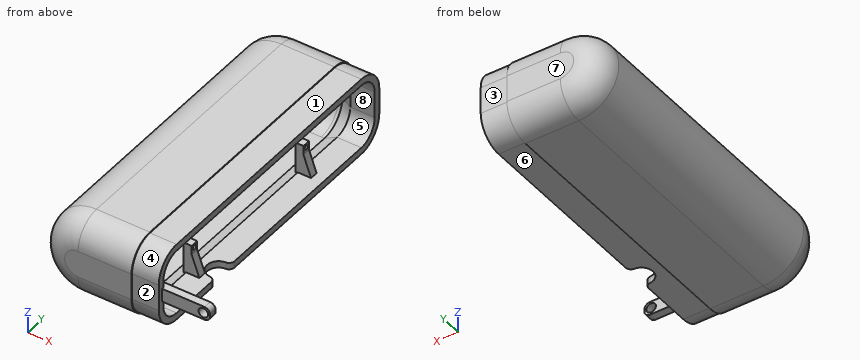
```python
from build123d import *
from OCP.BRepFilletAPI import BRepFilletAPI_MakeChamfer

# Parameters (mm, degrees)
BOSS_EXTRUDE1_DEPTH      = 76.2
FILLET1_R                = 12.7
SHELL1_T                 = -0.4
EXTRUDE_THIN1_DEPTH      = 12.7
EXTRUDE_THIN1_DEPTH_BACK = 6.35
CHAMFER1_SIZE            = 7.46
CHAMFER1_SIZE_2          = 3.96655236
SKETCH6_W                = 17.539309582
SKETCH6_H                = 3.81
SKETCH6_R                = 1.054294776
BOSS_EXTRUDE3_DEPTH      = 3.81
CHAMFER2_SIZE            = 10
CHAMFER2_SIZE2           = 3.639702343
SKETCH7_W                = 33.02
SKETCH7_H                = 6.35
BOSS_EXTRUDE4_DEPTH      = 3.81
CHAMFER3_SIZE            = 3.81
CHAMFER3_SIZE_2          = 4.231433681
SKETCH8_R                = 2.25
CUT_EXTRUDE1_DEPTH       = 160.403972974
FILLET2_R                = 2.54
SKETCH9_R                = 5.461
CUT_EXTRUDE2_DEPTH       = 104.511048806
FILLET3_R                = 2.54


with BuildPart() as part:
    # Sketch1 → Boss-Extrude1 (new, symmetric)
    with BuildSketch(Plane(origin=(0, 0, 0), x_dir=(1, 0, 0), z_dir=(0, 1, 0))):
        with BuildLine():
            Line((0, -19.05), (25.4, -19.05))
            Line((25.4, -19.05), (25.4, 19.05))
            Line((25.4, 19.05), (0, 19.05))
            ThreePointArc((0, 19.05), (-19.05, 0), (0, -19.05))
        make_face()
    extrude(amount=BOSS_EXTRUDE1_DEPTH, both=True)

    # Fillet1
    fillet1_edges = [part.edges().sort_by_distance(p)[0] for p in [
        (12.7, 76.2, -19.05),
        (-19.05, 76.2, 0),
        (12.7, -76.2, -19.05),
        (12.7, -76.2, 19.05),
        (-19.05, -76.2, 0),
        (12.7, 76.2, 19.05),
    ]]
    fillet(fillet1_edges, radius=FILLET1_R)

    # Shell1
    shell1_openings = [part.faces().sort_by_distance(p)[0] for p in [
        (25.4, 0, 0),
    ]]
    offset(amount=SHELL1_T, openings=shell1_openings, kind=Kind.INTERSECTION)

    # Sketch4 → Extrude-Thin1 (add, two sides: drawn at the far end of the back side and taken through both)
    with BuildSketch(Plane(origin=(25.4, 0, 0), x_dir=(0, 0, -1), z_dir=(1, 0, 0)).offset(-EXTRUDE_THIN1_DEPTH_BACK)):
        with BuildLine():
            Line((18.65, 63.5), (18.65, -63.5))
            ThreePointArc((18.65, -63.5), (15.047413409, -72.197413409), (6.35, -75.8))
            Line((6.35, -75.8), (-6.35, -75.8))
            ThreePointArc((-6.35, -75.8), (-15.047413409, -72.197413409), (-18.65, -63.5))
            Line((-18.65, -63.5), (-18.65, 63.5))
            ThreePointArc((-18.65, 63.5), (-15.047413409, 72.197413409), (-6.35, 75.8))
            Line((-6.35, 75.8), (6.35, 75.8))
            ThreePointArc((6.35, 75.8), (15.047413409, 72.197413409), (18.65, 63.5))
        make_face()
        with BuildLine():
            Line((15.475, 63.5), (15.475, -63.5))
            ThreePointArc((15.475, -63.5), (12.802349378, -69.952349378), (6.35, -72.625))
            Line((6.35, -72.625), (-6.35, -72.625))
            ThreePointArc((-6.35, -72.625), (-12.802349378, -69.952349378), (-15.475, -63.5))
            Line((-15.475, -63.5), (-15.475, 63.5))
            ThreePointArc((-15.475, 63.5), (-12.802349378, 69.952349378), (-6.35, 72.625))
            Line((-6.35, 72.625), (6.35, 72.625))
            ThreePointArc((6.35, 72.625), (12.802349378, 69.952349378), (15.475, 63.5))
        make_face(mode=Mode.SUBTRACT)
    extrude(amount=EXTRUDE_THIN1_DEPTH + EXTRUDE_THIN1_DEPTH_BACK)

    # Chamfer1
    # the kernel refuses this chamfer: 7.46, 3.96655236 mm, written as the material it takes off along each edge
    with BuildSketch(Plane(origin=(19.05, 63.5, -15.475), x_dir=(0.9998355423896509, 0, 0.01813527431257697), z_dir=(0, -1, 0))) as chamfer1_piece_1_section:
        Polygon((CHAMFER1_SIZE * 0.99983554239, -CHAMFER1_SIZE * 0.0181352743126), (-CHAMFER1_SIZE_2 * 0.0181352743135, -CHAMFER1_SIZE_2 * 0.999835542439), (0, 0), align=None)
    chamfer1_piece_1 = extrude(amount=127, mode=Mode.PRIVATE)
    chamfer1_piece_1 = split(chamfer1_piece_1, bisect_by=Plane(origin=(21.815261342, 60.108381876, -18.65), z_dir=(0, 0, 1)), keep=Keep.TOP, mode=Mode.PRIVATE)
    add(chamfer1_piece_1, mode=Mode.SUBTRACT)
    with BuildSketch(Plane(origin=(19.05, 63.5, -6.35), x_dir=(0, 1, 0), z_dir=(0, 0, 1))) as chamfer1_piece_2_section:
        Polygon((9.125, -CHAMFER1_SIZE), (9.125 + CHAMFER1_SIZE_2, 0), (9.125, 0), align=None)
    chamfer1_piece_2 = revolve(axis=Axis((19.05, 63.5, -6.35), (-1, 0, 0)), revolution_arc=90, mode=Mode.PRIVATE)
    chamfer1_piece_2 = chamfer1_piece_2 & Plane(origin=(21.967036343, 63.5, -6.35), x_dir=(0, 0, -1), z_dir=(-1, 0, 0)) * Cylinder(12.3, 53, mode=Mode.PRIVATE)
    add(chamfer1_piece_2, mode=Mode.SUBTRACT)
    with BuildSketch(Plane(origin=(19.05, -63.5, -6.35), x_dir=(0, 0, -1), z_dir=(0, 1, 0))) as chamfer1_piece_3_section:
        Polygon((9.125, -CHAMFER1_SIZE), (9.125 + CHAMFER1_SIZE_2, 0), (9.125, 0), align=None)
    chamfer1_piece_3 = revolve(axis=Axis((19.05, -63.5, -6.35), (-1, 0, 0)), revolution_arc=90, mode=Mode.PRIVATE)
    chamfer1_piece_3 = chamfer1_piece_3 & Plane(origin=(21.967036343, -63.5, -6.35), x_dir=(0, 0, -1), z_dir=(-1, 0, 0)) * Cylinder(12.3, 53, mode=Mode.PRIVATE)
    add(chamfer1_piece_3, mode=Mode.SUBTRACT)
    with BuildSketch(Plane(origin=(19.05, 72.625, 6.35), x_dir=(0.9998355423896509, -0.01813527431257697, 0), z_dir=(0, 0, -1))) as chamfer1_piece_4_section:
        Polygon((CHAMFER1_SIZE * 0.99983554239, -CHAMFER1_SIZE * 0.0181352743126), (-CHAMFER1_SIZE_2 * 0.0181352743135, -CHAMFER1_SIZE_2 * 0.999835542439), (0, 0), align=None)
    chamfer1_piece_4 = extrude(amount=12.7, mode=Mode.PRIVATE)
    chamfer1_piece_4 = split(chamfer1_piece_4, bisect_by=Plane(origin=(21.637658595, 75.8, 3.947497634), z_dir=(0, -1, 0)), keep=Keep.TOP, mode=Mode.PRIVATE)
    add(chamfer1_piece_4, mode=Mode.SUBTRACT)
    with BuildSketch(Plane(origin=(19.05, -72.625, -6.35), x_dir=(0.9998355423896509, 0.01813527431257697, 0), z_dir=(0, 0, 1))) as chamfer1_piece_5_section:
        Polygon((CHAMFER1_SIZE * 0.99983554239, -CHAMFER1_SIZE * 0.0181352743126), (-CHAMFER1_SIZE_2 * 0.0181352743135, -CHAMFER1_SIZE_2 * 0.999835542439), (0, 0), align=None)
    chamfer1_piece_5 = extrude(amount=12.7, mode=Mode.PRIVATE)
    chamfer1_piece_5 = split(chamfer1_piece_5, bisect_by=Plane(origin=(21.637658595, -75.8, -3.947497634), z_dir=(0, 1, 0)), keep=Keep.TOP, mode=Mode.PRIVATE)
    add(chamfer1_piece_5, mode=Mode.SUBTRACT)
    with BuildSketch(Plane(origin=(19.05, 63.5, 6.35), x_dir=(0, 0, 1), z_dir=(0, -1, 0))) as chamfer1_piece_6_section:
        Polygon((9.125, -CHAMFER1_SIZE), (9.125 + CHAMFER1_SIZE_2, 0), (9.125, 0), align=None)
    chamfer1_piece_6 = revolve(axis=Axis((19.05, 63.5, 6.35), (-1, 0, 0)), revolution_arc=90, mode=Mode.PRIVATE)
    chamfer1_piece_6 = chamfer1_piece_6 & Plane(origin=(21.967036343, 63.5, 6.35), x_dir=(0, 0, 1), z_dir=(1, 0, 0)) * Cylinder(12.3, 53, mode=Mode.PRIVATE)
    add(chamfer1_piece_6, mode=Mode.SUBTRACT)
    with BuildSketch(Plane(origin=(19.05, -63.5, 6.35), x_dir=(0, -1, 0), z_dir=(0, 0, -1))) as chamfer1_piece_7_section:
        Polygon((9.125, -CHAMFER1_SIZE), (9.125 + CHAMFER1_SIZE_2, 0), (9.125, 0), align=None)
    chamfer1_piece_7 = revolve(axis=Axis((19.05, -63.5, 6.35), (-1, 0, 0)), revolution_arc=90, mode=Mode.PRIVATE)
    chamfer1_piece_7 = chamfer1_piece_7 & Plane(origin=(21.967036343, -63.5, 6.35), x_dir=(0, 0, 1), z_dir=(1, 0, 0)) * Cylinder(12.3, 53, mode=Mode.PRIVATE)
    add(chamfer1_piece_7, mode=Mode.SUBTRACT)
    with BuildSketch(Plane(origin=(19.05, -63.5, 15.475), x_dir=(0.9998355423896509, 0, -0.01813527431257697), z_dir=(0, 1, 0))) as chamfer1_piece_8_section:
        Polygon((CHAMFER1_SIZE * 0.99983554239, -CHAMFER1_SIZE * 0.0181352743126), (-CHAMFER1_SIZE_2 * 0.0181352743135, -CHAMFER1_SIZE_2 * 0.999835542439), (0, 0), align=None)
    chamfer1_piece_8 = extrude(amount=127, mode=Mode.PRIVATE)
    chamfer1_piece_8 = split(chamfer1_piece_8, bisect_by=Plane(origin=(21.815261342, -60.108381876, 18.65), z_dir=(0, 0, -1)), keep=Keep.TOP, mode=Mode.PRIVATE)
    add(chamfer1_piece_8, mode=Mode.SUBTRACT)

    # Sketch6 → Boss-Extrude3 (add)
    # profile 1 of 2: a face of its own
    with BuildSketch(Plane(origin=(25.4, 0, 0), x_dir=(0, 0, -1), z_dir=(1, 0, 0))):
        with Locations((9.880345209, 38.431496192)):
            Rectangle(SKETCH6_W, SKETCH6_H)
        with Locations(Location((3.015690418, 38.431496192, 0), (0, 0, 180))):
            Circle(SKETCH6_R, mode=Mode.SUBTRACT)
    # profile 2 of 2: a face of its own
    with BuildSketch(Plane(origin=(25.4, 0, 0), x_dir=(0, 0, -1), z_dir=(1, 0, 0))):
        with Locations((9.880345209, -38.410993514)):
            Rectangle(SKETCH6_W, SKETCH6_H)
        with Locations(Location((3.015690418, -38.410993514, 0), (0, 0, 180))):
            Circle(SKETCH6_R, mode=Mode.SUBTRACT)
    extrude(amount=BOSS_EXTRUDE3_DEPTH)

    # Chamfer2: one chamfer whose edges measure the first distance from different faces: ONE call of the kernel's chamfer builder (chamfer() names one face for all edges)
    chamfer2_edges_1 = [part.edges().sort_by_distance(p)[0] for p in [
        (29.21, -38.410993514, -15.475),
    ]]
    chamfer2_side_1 = [part.faces().sort_by_distance(p)[0] for p in [
        (29.21, -38.410993514, -8.652510406),
    ]]
    chamfer2_edges_2 = [part.edges().sort_by_distance(p)[0] for p in [
        (29.21, 38.431496192, -15.475),
    ]]
    chamfer2_side_2 = [part.faces().sort_by_distance(p)[0] for p in [
        (29.21, 38.431496192, -8.652510406),
    ]]
    chamfer2 = BRepFilletAPI_MakeChamfer(part.part.solid().wrapped)
    for e in chamfer2_edges_1:
        chamfer2.Add(CHAMFER2_SIZE, CHAMFER2_SIZE2, e.wrapped, chamfer2_side_1[0].wrapped)  # the first distance lies on this face
    for e in chamfer2_edges_2:
        chamfer2.Add(CHAMFER2_SIZE, CHAMFER2_SIZE2, e.wrapped, chamfer2_side_2[0].wrapped)  # the first distance lies on this face
    add(Compound.cast(chamfer2.Shape()), mode=Mode.REPLACE)

    # Sketch7 → Boss-Extrude4 (add)
    with BuildSketch(Plane(origin=(0, -73.66, 0), x_dir=(1, 0, 0), z_dir=(0, 1, 0))):
        with Locations((44.45, 0)):
            Rectangle(SKETCH7_W, SKETCH7_H)
    extrude(amount=BOSS_EXTRUDE4_DEPTH)

    # Chamfer3
    # the kernel refuses this chamfer: 4.231433681, 3.81 mm, written as the material it takes off along each edge
    with BuildSketch(Plane(origin=(27.94, -69.85, -3.175), x_dir=(-0.03204434000819545, -0.9994864482690294, 0), z_dir=(0, 0, 1))) as chamfer3_piece_1_section:
        Polygon((CHAMFER3_SIZE * 0.999486448269, CHAMFER3_SIZE * 0.0320443400082), (-CHAMFER3_SIZE_2 * 0.032044340012, CHAMFER3_SIZE_2 * 0.999486448387), (0, 0), align=None)
    chamfer3_piece_1 = extrude(amount=6.35, mode=Mode.PRIVATE)
    chamfer3_piece_1 = split(chamfer3_piece_1, bisect_by=Plane(origin=(28.695678786, -72.625, -2.695594609), z_dir=(0, 1, 0)), keep=Keep.TOP, mode=Mode.PRIVATE)
    add(chamfer3_piece_1, mode=Mode.SUBTRACT)

    # Sketch8 → Cut-Extrude1 (cut, through all)
    with BuildSketch(Plane(origin=(0, -69.85, 0), x_dir=(1, 0, 0), z_dir=(0, 1, 0))):
        with Locations(Location((57.785, 0, 0), (0, 0, 270))):
            Circle(SKETCH8_R)
    extrude(amount=-CUT_EXTRUDE1_DEPTH, mode=Mode.SUBTRACT)

    # Fillet2
    fillet2_edges = [part.edges().sort_by_distance(p)[0] for p in [
        (60.96, -71.755, -3.175),
        (60.96, -71.755, 3.175),
    ]]
    fillet(fillet2_edges, radius=FILLET2_R)

    # Sketch9 → Cut-Extrude2 (cut, through all)
    with BuildSketch(Plane.XY.offset(-15.475)):
        with Locations((36.068, -31.75)):
            Circle(SKETCH9_R)
    extrude(amount=-CUT_EXTRUDE2_DEPTH, mode=Mode.SUBTRACT)

    # Fillet3
    fillet3_edges = [part.edges().sort_by_distance(p)[0] for p in [
        (38.1, -26.681124681, -17.0625),
        (38.1, -36.818875319, -17.0625),
    ]]
    fillet(fillet3_edges, radius=FILLET3_R)


solid = part.part
```
The model under review builds one solid part; all positions refer to its coordinate system, in mm. Face numbers are marked on the shaded views. A direction names the side the tool comes from. Give positions to 0.01 mm unless a question says otherwise; leave off trailing zeros. Order: outer loops, then holes, each group sorted by start corner. A loop starts at its lowest first (then second) coordinate and runs counter-clockwise, first axis right, second up. Notation, with made-up numbers: (53, 35.25) - (90, 35.25) arc R29 ccw to (90, 62.25) - close; hole circle Ø1 at (40.25, -30). An arc over 180 degrees is marked (long way). Use CSV: the item, a comma, the result in double quotes. Start each with the question number.
Q1. To check wall thickness, follow line 1 along Z through (x, y) = (31, -19) (3 decimals); line 2 along Y through (x, z) = (12.5, 1.5). State the ranges of each line that lie inside material, in increasing order. Write a range as [from, to].
Q2. Clearance check with flat-ended pins moving along their axes: pin 1 Ø9.5 at (x, y) = (33, -1.5) entering from +Z; pin 2 Ø1.3 at (y, z) = (38.43, -3.02) entering from -X; pin 3 Ø6 at (x, z) = (27.5, -9) entering from -Y; pin 4 Ø14 at (x, y) = (32, 9.5) entering from +Z. State where each tip first meets the part, or that it passes through.
Q3. The part is to be moulded in two halves that separate along Z. For the marked faces 6, 7 and 8, say which applies: +Z half, -Z half, draft (parallel to the pull), parting line (faces both ways), or undercut.
Q4. We need section B-B, the plane y = -31.75. Write out the cut boundary in (x, z) (3 decimals).
Q5. We need section A-A, the plane x = 1.5. Write out the cut boundary in (y, z).
Q6. Tool access review of the marked faces 1, 2, 3, 4 and 5: name each direction out of +Z, -Z, +X, -X, +Y, -Y from which nothing blocks a thin tool from reaching the whole face with its end or side.
Q7. We need section C-C, the plane z = -12.5. State how many separate pieces and enclosed holes the cut face has, and give its area (3 significant figures).
Q8. We need section D-D, the plane y = 4.5. Write out the cut boundary in (x, z) (3 decimals), and give its area (3 significant figures).
Outcome:
1,line 1,"z = [-18.65, -15.475], [15.475, 18.65]"
1,line 2,"y = [-76.2, -75.8], [75.8, 76.2]"
2,pin 1,"stops at z = 18.65"
2,pin 2,"stops at x = -18.9"
2,pin 3,"stops at y = -76.19"
2,pin 4,"stops at z = 19.05"
3,face 6,"-Z half"
3,face 7,"draft"
3,face 8,"undercut"
4,outline,"(0, -19.05) - (25.4, -19.05) - (25.4, -18.65) - (30.607, -18.65) - (30.607, -15.475) - (26.51, -15.475) - (20.539, -18.65) - (0, -18.65) arc R18.65 cw to (0, 18.65) - (20.539, 18.65) - (26.51, 15.475) - (38.1, 15.475) - (38.1, 18.65) - (25.4, 18.65) - (25.4, 19.05) - (0, 19.05) arc R19.05 ccw to start"
5,outline,"(-76.2, -6.35) arc R12.7 ccw to (-63.5, -19.05) - (63.5, -19.05) arc R12.7 ccw to (76.2, -6.35) - (76.2, 6.35) arc R12.7 ccw to (63.5, 19.05) - (-63.5, 19.05) arc R12.7 ccw to (-76.2, 6.35) - close; hole (-75.8, -6.35) arc R12.3 ccw to (-63.5, -18.65) - (63.5, -18.65) arc R12.3 ccw to (75.8, -6.35) - (75.8, 6.35) arc R12.3 ccw to (63.5, 18.65) - (-63.5, 18.65) arc R12.3 ccw to (-75.8, 6.35) - close"
6,face 1,"+Z, +X, +Y, -Y"
6,face 2,"+Z, -Z, +X, -Y"
6,face 3,"+Z, -Z, +X, +Y"
6,face 4,"+Z, +X, -Y"
6,face 5,"+X"
7,separate pieces,"3"
7,enclosed holes,"0"
7,area,"273 mm^2"
8,outline,"(0, -19.05) - (25.4, -19.05) - (25.4, -18.65) - (38.1, -18.65) - (38.1, -15.475) - (26.51, -15.475) - (20.539, -18.65) - (0, -18.65) arc R18.65 cw to (0, 18.65) - (20.539, 18.65) - (26.51, 15.475) - (38.1, 15.475) - (38.1, 18.65) - (25.4, 18.65) - (25.4, 19.05) - (0, 19.05) arc R19.05 ccw to start"
8,area,"137 mm^2"
